Geometry check sheet. Reference: the model listing, model coordinates, mm. A direction names the side the tool comes from. Round coordinates to 2 decimals unless told otherwise and drop trailing zeros. Loops run counter-clockwise (first coordinate to the right, second up) from the corner with the lowest first, then second, coordinate; pieces in that order, holes last. Notation, with made-up numbers: (43, 76.5) - (59, 76.5) arc R15 cw to (59, 98.5) - close; hole circle Ø1 at (17.5, 68.5). An arc over 180 degrees is marked (long way). Answer in a Markdown table with one row per item. Add a question column.
```python
from build123d import *

# Parameters (mm, degrees)
F4_R = 2
F5_R = 2
F6_R = 2


# Not quite as in the source:
# - a fillet or chamfer that OpenCascade refuses, or shapes differently, is made with other operations: its cross-section is extruded or revolved along the edge and cut away or added


with BuildPart() as f1:
    # F0 (on Front) → F1 (revolve)
    with BuildSketch(Plane.XZ):
        with BuildLine():
            Line((0, 31), (0, 0))
            Line((0, 0), (9, 0))
            Line((9, 0), (9, 5))
            Line((9, 5), (8.5, 5))
            Line((8.5, 5), (8.5, 8))
            Line((8.5, 8), (7, 8))
            Line((7, 8), (5.5, 15.5))
            Line((5.5, 15.5), (4.25, 15.5))
            Line((4.25, 15.5), (4.25, 18))
            Line((4.25, 18), (6, 18))
            Line((6, 18), (4, 22))
            Line((4, 22), (4.5, 22))
            add(Edge.make_bspline(
                [(4.5, 31), (5, 29.5), (6, 26.5), (5, 23.5), (4.5, 22)],
                knots=[0, 0, 0, 0, 0.5, 1, 1, 1, 1], degree=3))
            Line((4.5, 31), (0, 31))
        make_face()
    revolve(axis=Axis((0, 0, 15.5), (0, 0, 1)))

    # F2: fillet of radius 2 on 1 edges, made by hand

    # F2_s1 → F2_t2 (revolve)
    with BuildSketch(Plane.XZ):
        with BuildLine():
            ThreePointArc((5.5, 15.5), (4.5916876048, 16.236015633), (4.25, 17.3540496218))
            Line((4.25, 17.3540496218), (4.25, 15.5))
            Line((4.25, 15.5), (5.5, 15.5))
        make_face()
    revolve(axis=Axis((0, 0, 15.5), (0, 0, 1)))

    # F3: fillet of radius 8 on 1 edges, made by hand

    # F3_s1 → F3_t2 (revolve)
    with BuildSketch(Plane.XZ):
        with BuildLine():
            ThreePointArc((8.5, 8), (6.9960478639, 9.9399549841), (6.1510825053, 12.2445874734))
            Line((6.1510825053, 12.2445874734), (5.9941895972, 12.2132088918))
            Line((5.9941895972, 12.2132088918), (6.8431070919, 7.9686214184))
            Line((6.8431070919, 7.9686214184), (7, 7.84))
            ThreePointArc((7, 7.84), (7.75, 7.84), (8.3900854418, 7.8837296689))
            Line((8.3900854418, 7.8837296689), (8.5, 8))
        make_face()
    revolve(axis=Axis((0, 0, 8), (0, 0, 1)))

    # F4
    f4_edges = [f1.edges().sort_by_distance(p)[0] for p in [
        (-5.5, 0, 15.5),
    ]]
    fillet(f4_edges, radius=F4_R)

    # F5
    f5_edges = [f1.edges().sort_by_distance(p)[0] for p in [
        (-8.5, 0, 8),
    ]]
    fillet(f5_edges, radius=F5_R)

    # F6
    f6_edges = [f1.edges().sort_by_distance(p)[0] for p in [
        (-4.5, 0, 31),
    ]]
    fillet(f6_edges, radius=F6_R)

    # F7: chamfer of 1.5 x 0.5 on 1 edges, made by hand

    # F7_s1 → F7_t2 (revolve, cut)
    with BuildSketch(Plane.XZ):
        Polygon((5.7763932023, 18.4472135955), (4.5, 18), (6, 18), align=None)
    revolve(axis=Axis((0, 0, 18), (0, 0, 1)), mode=Mode.SUBTRACT)


solid = f1.part
```
Q1. Depth check by flat-ended pin: P1, Ø7, axis at x = 0, y = -0.5, coming from the -Z side; P2, Ø5, axis at x = -0.5, z = 12, coming from the -Y side; P3, Ø10, axis at x = 6.5, z = 16, coming from the -Y side; P4, Ø6, axis at x = 5, y = 4, coming from the +Z side. Enter the tip coordinate at first touch or a pass-through.
Q2. Scan lines: line 1 (Z direction, x = -3.25, y = -3); line 2 (Z direction, x = -7.75, y = 4.5); line 3 (Y direction, x = -0.5, z = 7). Record each from-to range of solid material in increasing order. Write a range as from..to.
Q3. Cross-section at A-A, the plane z = 14. Enter the section's corners in (x, y), plus the area to 3 significant figures.
Q4. Release check for a two-part mould opening along Z. For faces 1 (the flat face through (0, 0, 31)), 2 (the flat face through (0, 0, 0)), 3 (the flat face through (3, -3, 22)) record: +Z half, -Z half, draft (parallel to the pull), parting line (faces both ways), or undercut.
Q5. Set-up check for faces 4 (the cylindrical face through (-6.265, 5.745, 6.113)), 5 (the cylindrical face through (-1.172, 8.923, 2.535)), 6 (the cylindrical face through (2.285, 3.584, 17.682)): record each of +Z, -Z, +X, -X, +Y, -Y from which the full face is reachable in a straight line by a thin tool's end or side.
Check sheet entries:
| question | item | result |
|---|---|---|
| 1 | P1 | z = 0 |
| 1 | P2 | y = -7.25 |
| 1 | P3 | y = -5.49 |
| 1 | P4 | z = 30.97 |
| 2 | line 1 | 0..16.54, 18..21.15, 22..30.45 |
| 2 | line 2 | 0..5 |
| 2 | line 3 | -8.49..8.49 |
| 3 | outline | circle Ø11.6 at (0, 0) |
| 3 | area | 106 mm² |
| 4 | face 1 | +Z half |
| 4 | face 2 | -Z half |
| 4 | face 3 | undercut |
| 5 | face 4 | +Z |
| 5 | face 5 | +Z, -Z |
| 5 | face 6 | none |
